Answer from the drawing. Dimensions are ordinates in mm from the lowest x, y and z of the part. Give positions to 0.01 mm unless a question says otherwise; leave off trailing zeros. Loops run counter-clockwise (first coordinate to the right, second up) from the corner with the lowest first, then second, coordinate; pieces in that order, holes last. Notation, with made-up numbers: (19, 61.5) - (54, 61.5) arc R12 ccw to (54, 74.5) - close; hole circle Ø10 at (-8, 72.5). An arc over 180 degrees is marked (long way). One line per item, written item: value.
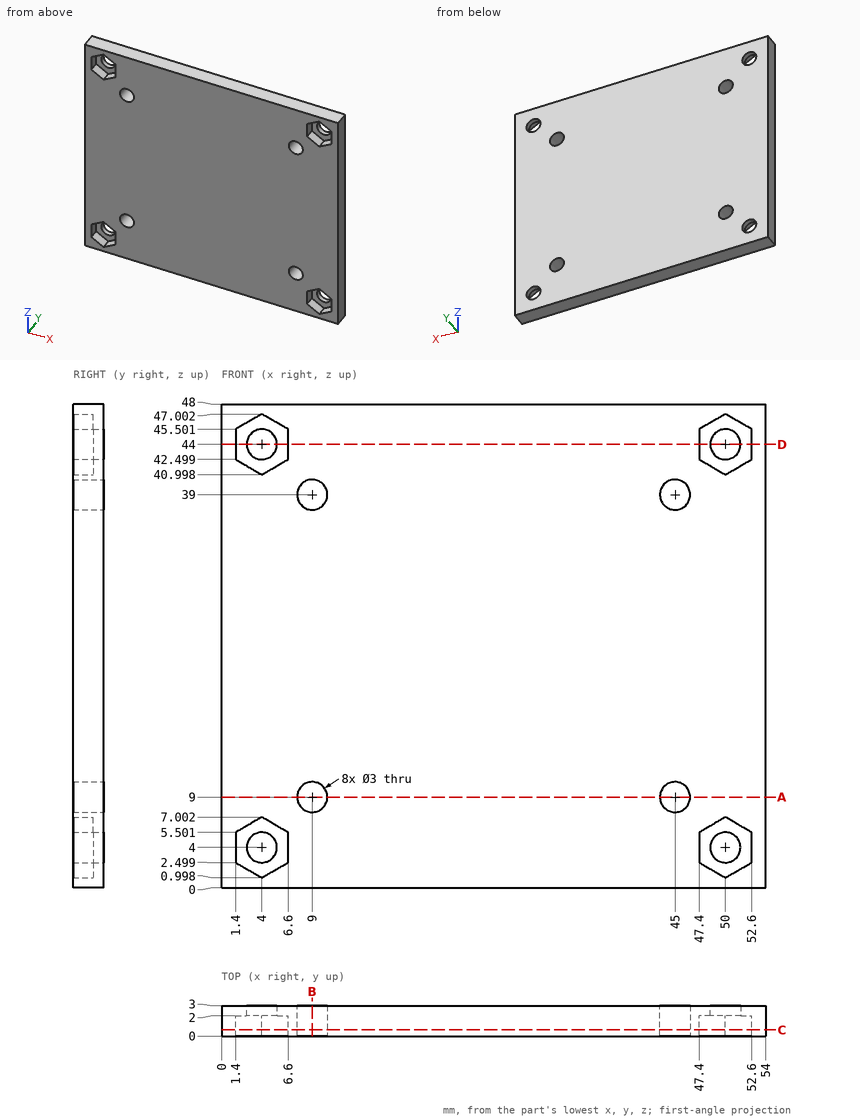
1. Section D-D (z = 44) is taken. Write down the section's boundary in (x, y), and give its area (3 significant figures).
Output:
outline: (0, 0) - (1.4, 0) - (1.4, 2) - (2.5, 2) - (2.5, 3) - (0, 3) - close; (5.5, 2) - (6.6, 2) - (6.6, 0) - (47.4, 0) - (47.4, 2) - (48.5, 2) - (48.5, 3) - (5.5, 3) - close; (51.5, 2) - (52.6, 2) - (52.6, 0) - (54, 0) - (54, 3) - (51.5, 3) - close
area: 135 mm²
2. Section B-B (x = 9) is taken. Write down the section's boundary in (y, z), and give its area (3 significant figures).
Output:
outline: (0, 0) - (3, 0) - (3, 7.5) - (0, 7.5) - close; (0, 10.5) - (3, 10.5) - (3, 37.5) - (0, 37.5) - close; (0, 40.5) - (3, 40.5) - (3, 48) - (0, 48) - close
area: 126 mm²
3. Section A-A (z = 9) is taken. Write down the section's boundary in (x, y), and give its area (3 significant figures).
Output:
outline: (0, 0) - (7.5, 0) - (7.5, 3) - (0, 3) - close; (10.5, 0) - (43.5, 0) - (43.5, 3) - (10.5, 3) - close; (46.5, 0) - (54, 0) - (54, 3) - (46.5, 3) - close
area: 144 mm²
4. Find the intervals of material crossed by line 1 along X through (y, z) = (0.75, 4.5); line 2 along Z through (x, y) = (50, 2.45); line 3 along Z through (x, y) = (3.5, 0.4), in increasing order.
Output:
line 1: x = 0 to 1.4, 6.6 to 47.4, 52.6 to 54
line 2: z = 0 to 2.5, 5.5 to 42.5, 45.5 to 48
line 3: z = 0 to 1.29, 6.71 to 41.29, 46.71 to 48
5. Section C-C (y = 0.6) is taken. Count the separate pieces of the cut face and the enclosed holes in it, and give its area (3 significant figures).
Output:
separate pieces: 1
enclosed holes: 8
area: 2,470 mm²
6. A flat-ended cylindrical pin translates along its axis: pin 1 Ø1.6 at (x, z) = (49.5, 5.5) entering from -Y. Find the tip coordinate at first contact, or state that the pin passes through.
Output:
pin 1: stops at y = 2
